```python
from build123d import *

# Parameters (mm, degrees)
DWIRE007_W       = 1.028705
DWIRE007_H       = 1.001781
EXTRUDE007_DEPTH = 9
ARRAY001_Y_COUNT = 20
ARRAY001_Y_PITCH = 2
DWIRE016_W       = 0.7
DWIRE016_H       = 38.839707
EXTRUDE019_DEPTH = 9
DWIRE017_W       = 4.407525
DWIRE017_H       = 8.059332
EXTRUDE020_DEPTH = 14


with BuildPart() as obj1:
    # DWire007 → Extrude007 (new body)
    with BuildSketch(Plane.XY):
        with Locations((0.514352, 0.500891)):
            Rectangle(DWIRE007_W, DWIRE007_H)
    extrude(amount=EXTRUDE007_DEPTH)


with BuildPart() as obj1_1:
    # Extrude007 placement: moved
    add(obj1.part.moved(Location((0, 0, 6))))

    # Array001 Y: obj1 ×20


with BuildPart() as obj1_2:
    add(obj1_1.part)
    with Locations(*[(0, i * ARRAY001_Y_PITCH, 0) for i in range(1, ARRAY001_Y_COUNT)]):
        add(obj1_1.part)


with BuildPart() as obj2:
    # DWire016 → Extrude019 (new body)
    with BuildSketch(Plane.XY):
        with Locations((-0.05, 19.419853)):
            Rectangle(DWIRE016_W, DWIRE016_H)
    extrude(amount=EXTRUDE019_DEPTH)


with BuildPart() as obj2_1:
    # Extrude019 placement: moved
    add(obj2.part.moved(Location((0, 0, 6))))

    # Fusion002: union obj1
    add(obj1_2.part)


with BuildPart() as obj3:
    # DWire017 → Extrude020 (new body)
    with BuildSketch(Plane.XY):
        with Locations((0.16035, 17.61238)):
            Rectangle(DWIRE017_W, DWIRE017_H)
    extrude(amount=EXTRUDE020_DEPTH)

    # Cut015: cut obj2
    add(obj2_1.part, mode=Mode.SUBTRACT)


solid = obj3.part
```
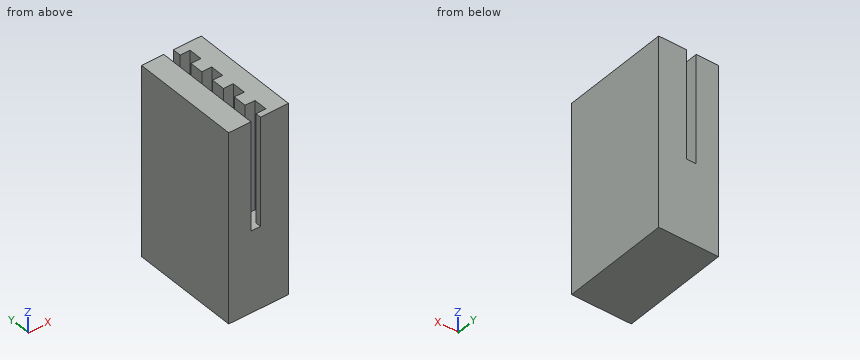
Geometry: final body of the model. Coordinates: model frame, mm. Round coordinates to 2 decimals unless told otherwise and drop trailing zeros. Loops run counter-clockwise (first coordinate to the right, second up) from the corner with the lowest first, then second, coordinate; pieces in that order, holes last. Notation, with made-up numbers: (47, 40.5) -> (57, 40.5) arc R16 ccw to (57, 55.5) -> close; hole circle Ø3 at (52, 7.5). An arc over 180 degrees is marked (long way). Use one line per item in the form item = value. Start each with the question number.
1) Section A-A on z = 8.5. Output: boundary loops of the cut face in (x, y), then the cut area to 3 significant figures.
2) Line query: L1, parallel to Y at x = 0.95, z = 6.5; L2, parallel to X at y = 21.25, z = 8; L3, parallel to X at y = 14.5, z = 12.75. Output: solid intervals per line, ascending.
3) Section B-B on y = 16.5. Output: boundary loops of the cut face in (x, z).
4) Section C-C on y = 15.25. Output: boundary loops of the cut face in (x, z), then the cut area to 3 significant figures.
Response:
q1.outline = (-2.04, 13.58) -> (-0.4, 13.58) -> (-0.4, 21.64) -> (-2.04, 21.64) -> close; (0.3, 13.58) -> (2.36, 13.58) -> (2.36, 21.64) -> (0.3, 21.64) -> (0.3, 21) -> (1.03, 21) -> (1.03, 20) -> (0.3, 20) -> (0.3, 19) -> (1.03, 19) -> (1.03, 18) -> (0.3, 18) -> (0.3, 17) -> (1.03, 17) -> (1.03, 16) -> (0.3, 16) -> (0.3, 15) -> (1.03, 15) -> (1.03, 14) -> (0.3, 14) -> close
q1.area = 27.0 mm^2
q2.L1 = 13.58 to 14, 15 to 16, 17 to 18, 19 to 20, 21 to 21.64
q2.L2 = -2.04 to -0.4, 0.3 to 2.36
q2.L3 = -2.04 to -0.4, 1.03 to 2.36
q3.outline = (-2.04, 0) -> (2.36, 0) -> (2.36, 14) -> (1.03, 14) -> (1.03, 6) -> (-0.4, 6) -> (-0.4, 14) -> (-2.04, 14) -> close
q4.outline = (-2.04, 0) -> (2.36, 0) -> (2.36, 14) -> (0.3, 14) -> (0.3, 6) -> (-0.4, 6) -> (-0.4, 14) -> (-2.04, 14) -> close
q4.area = 56.1 mm^2
